Input: part model. Units: mm. Frame: model coordinates. Face numbers are marked on the shaded views. Coordinates: 2 decimals unless noted, no trailing zeros. Order: outer loops, then holes, each group sorted by start corner. A loop starts at its lowest first (then second) coordinate and runs counter-clockwise, first axis right, second up. Notation, with made-up numbers: M 73.25,29 L 99.25,29 A17 ccw 99.25,58 Z; hole C 72,37 d11. An arc over 180 degrees is marked long. Answer in a Markdown table with one row per item.
from build123d import *

# Parameters (mm, degrees)
F0_W     = 85.725
F0_H     = 76.2
F1_DEPTH = 19.05
F2_T     = -3.175
F4_DEPTH = 15.875
F6_DEPTH = 3.175
F7_R     = 3.175
F8_R     = 12.7


with BuildPart() as f1:
    # F0 (on Front) → F1 (new body)
    with BuildSketch(Plane.XZ):
        with Locations((42.8625, 38.1)):
            Rectangle(F0_W, F0_H)
    extrude(amount=F1_DEPTH)

    # F2
    f2_openings = [f1.faces().sort_by_distance(p)[0] for p in [
        (42.8625, -9.525, 76.2),
    ]]
    offset(amount=F2_T, openings=f2_openings)

    # F3 (on face) → F4 (cut, through all)
    with BuildSketch(Plane.XZ.offset(19.05)):
        Polygon((42.8625, 76.2), (19.05, 76.2), (19.05, 19.05), (33.3375, 19.05), (33.3375, 0), (42.8625, 0), align=None)
        Polygon((66.675, 76.2), (42.8625, 76.2), (42.8625, 0), (52.3875, 0), (52.3875, 19.05), (66.675, 19.05), align=None)
    extrude(amount=-F4_DEPTH, mode=Mode.SUBTRACT)

    # F5 (on face) → F6 (join, through all)
    with BuildSketch(Plane(origin=(0, 0, 0), x_dir=(-1, 0, 0), z_dir=(0, 1, 0))):
        with BuildLine():
            Line((-73.025, 76.2), (-12.7, 76.2))
            ThreePointArc((-12.7, 76.2), (-42.8625, 96.2271509033), (-73.025, 76.2))
        make_face()
    extrude(amount=-F6_DEPTH)

    # F7
    f7_edges = [f1.edges().sort_by_distance(p)[0] for p in [
        (3.175, -3.175, 39.6875),
        (3.175, -15.875, 39.6875),
        (12.7, -1.5875, 76.2),
        (73.025, -1.5875, 76.2),
        (82.55, -3.175, 39.6875),
        (82.55, -15.875, 39.6875),
        (66.675, -17.4625, 19.05),
        (19.05, -17.4625, 19.05),
        (18.25625, -3.175, 3.175),
        (3.175, -9.525, 3.175),
        (18.25625, -15.875, 3.175),
        (67.46875, -3.175, 3.175),
        (67.46875, -15.875, 3.175),
        (82.55, -9.525, 3.175),
        (85.725, -19.05, 38.1),
        (85.725, 0, 38.1),
        (0, 0, 38.1),
        (0, -19.05, 38.1),
        (0, -9.525, 0),
        (69.05625, -19.05, 0),
        (16.66875, -19.05, 0),
        (85.725, -9.525, 0),
    ]]
    fillet(f7_edges, radius=F7_R)

    # F8
    f8_edges = [f1.edges().sort_by_distance(p)[0] for p in [
        (19.05, -17.4625, 76.2),
        (66.675, -17.4625, 76.2),
        (52.3875, -17.4625, 19.05),
        (33.3375, -17.4625, 19.05),
    ]]
    fillet(f8_edges, radius=F8_R)


solid = f1.part
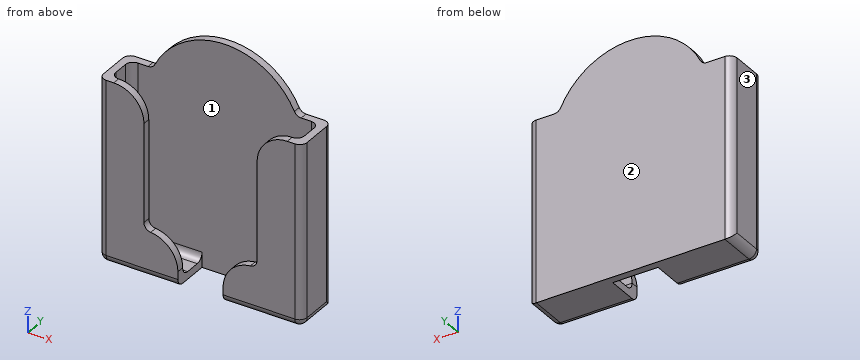
1) Mould query, pull axis Y, two halves, no side actions, for the marked faces 1, 2 and 3. Classes: +Y half, -Y half, draft (parallel to the pull), parting line (faces both ways), or undercut.
Resolved:
| item | result |
|---|---|
| face 1 | undercut |
| face 2 | +Y half |
| face 3 | draft |
2) Cut plane C-C, the plane x = 17.5. Output: boundary loops of the cut face in (y, z) (3 decimals).
Resolved:
| item | result |
|---|---|
| outline | M -19.05,3.175 A3.175 ccw -15.875,0 L 0,0 L 0,84.184 L -3.175,84.184 L -3.175,6.35 A3.175 cw -6.35,3.175 L -12.7,3.175 A3.175 cw -15.875,6.35 L -15.875,69.58 L -19.05,69.58 Z |
3) Contact query for flat-ended pins moving along their axis: pin 1 (1.9 mm diameter, centred on y = -10, z = 2, fed in from -X); pin 2 (5 mm diameter, centred on x = 24, y = -6.5, fed in from +Z) (3 decimals); pin 3 (5 mm diameter, centred on x = 71, y = -9.5, fed in from +Z) (3 decimals). Output: stop coordinate, or through.
Resolved:
| item | result |
|---|---|
| pin 1 | stops at x = 0.01 |
| pin 2 | stops at z = 4.215 |
| pin 3 | stops at z = 3.175 |
4) Material intervals for probe 1 along X at (y, z) = (-12.5, 62.5) (3 decimals); probe 2 along X at (y, z) = (-6, 62.5) (3 decimals); probe 3 along Y at (x, z) = (64, 16.5) (3 decimals), sorted ascending.
Resolved:
| item | result |
|---|---|
| probe 1 | x = 0 to 3.175, 82.55 to 85.725 |
| probe 2 | x = 0 to 3.194, 82.531 to 85.725 |
| probe 3 | y = -19.05 to -15.875, -3.175 to 0 |
5) Cut plane B-B, the plane z = 35. Output: boundary loops of the cut face in (x, y) (3 decimals), and give its area (3 significant figures).
Resolved:
| item | result |
|---|---|
| outline | M 0,-15.875 A3.175 ccw 3.175,-19.05 L 19.05,-19.05 L 19.05,-15.875 L 6.35,-15.875 A3.175 cw 3.175,-12.7 L 3.175,-6.35 A3.175 cw 6.35,-3.175 L 79.375,-3.175 A3.175 cw 82.55,-6.35 L 82.55,-12.7 A3.175 cw 79.375,-15.875 L 66.675,-15.875 L 66.675,-19.05 L 82.55,-19.05 A3.175 ccw 85.725,-15.875 L 85.725,-3.175 A3.175 ccw 82.55,0 L 3.175,0 A3.175 ccw 0,-3.175 Z |
| area | 474 mm2 |
